Can you work these out from the model? Positions are in its coordinate system, mm. Face numbers are marked on the shaded views. A direction names the side the tool comes from. Give positions to 0.01 mm unless a question says otherwise; leave off trailing zeros. Order: outer loops, then holes, each group sorted by start corner. A loop starts at its lowest first (then second) coordinate and runs counter-clockwise, first axis right, second up.
Item 1: I want a section at A-A, the plane x = 9. Write out the boundary of the cut face in (y, z).
Item 2: I'm going to push flat-ended pins straight in: pin 1 Ø4 at (y, z) = (9.5, 48.5) entering from +X; pin 2 Ø3 at (y, z) = (9.5, 12) entering from +X; pin 3 Ø8 at (y, z) = (9, 37) entering from +X. Where does each tip first touch, or does it pass through?
Item 3: I want a section at C-C, the plane z = 34. Write out the boundary of the cut face in (x, y), then the cut area to 3 significant figures.
Item 4: If I drill on line 1 along X through (y, z) = (-23.85, 2.5); line 2 along Z through (x, y) = (-9, -23.9); line 3 along Y through (x, z) = (-7, 44.5), over which ranges is the centre line in solid material (lowest first)?
Item 5: If we mould it in two halves opening along Y, with no side actions, what happens to the marked faces 1, 2 and 3? For each: +Y half, -Y half, draft (parallel to the pull), parting line (faces both ways), or undercut.
Item 6: I want a section at B-B, the plane z = 2.5. Count the separate pieces of the cut face and the enclosed holes in it, then the cut area to 3 significant figures.
Item 7: Which directions (+Z, -Z, +X, -X, +Y, -Y) give clear straight access to the entire face, cutting with the end or side of a thin tool? Please do the marked faces 4 and 5.
Item 8: I want a section at D-D, the plane y = 19. Write out the boundary of the cut face in (x, z).
Autodesk Inventor part; units mm, degrees
ref_plane "YZ Plane" through (0, 0, 0) normal (1, 0, 0) x (0, 1, 0)
ref_plane "XZ Plane" through (0, 0, 0) normal (0, 1, 0) x (-1, 0, 0)
ref_plane "XY Plane" through (0, 0, 0) normal (0, 0, 1) x (1, 0, 0)
sketch "Sketch1" plane through (0, 0, 0) normal (0, 0, 1) x (1, 0, 0)
  circle A0 centre (0, 0) radius 28.8
  line L0 (-50, 23.8) -> (50, 23.8)
  line L1 (50, 23.8) -> (50, -23.8)
  line L2 (50, -23.8) -> (-50, -23.8)
  line L3 (-50, -23.8) -> (-50, 23.8)
  point P0 (50, 0)
  point P1 (0, 23.8)
  point P2 (-16.217275, -23.8)
  point P3 (16.217275, -23.8)
  point P4 (16.217275, 23.8)
  point P5 (-16.217275, 23.8)
  dimension "d0" = 57.6
  dimension "d1" = 47.6
  dimension "d2" = 100
sketch "Sketch1 outline for Extrusion1" plane through (0, 0, 0) normal (0, 0, 1) x (1, 0, 0)
  line L0 (-16.217275, -23.8) -> (16.217275, -23.8)
  arc A0 (-16.217275, 23.8) -> (-16.217275, -23.8) centre (0, 0) ccw
  line L1 (16.217275, 23.8) -> (-16.217275, 23.8)
  arc A1 (16.217275, -23.8) -> (16.217275, 23.8) centre (0, 0) ccw
extrude "Extrusion1" add sketch "Sketch1 outline for Extrusion1" along normal blind 80
fillet "Fillet1" radius 1 4 edges at (-16.2173, 23.8, 40) (16.2173, 23.8, 40) (16.2173, -23.8, 40) (-16.2173, -23.8, 40)
thicken "Thicken1" operation add thickness 0.2 both sides no extend neighbours no toward (0, 1, 0) faces at (5.301991, 23.8, 26.666667) (-16.040924, 23.790852, 26.666667) (-27.332956, -9.074665, 53.333333) (16.237959, 23.743284, 26.666667) (28.430873, 4.596242, 53.333333) (16.362219, -23.689854, 26.666667) (-5.301991, -23.8, 26.666667) (-16.362219, -23.689854, 26.666667)
shell "Shell1" thickness 0.2 removed faces 2 at (-5.301991, -8, 80) at (-5.301991, -8, 0)
sketch "Sketch2" plane through (-19.580613, 24, 0) normal (0, 1, 0) x (1, 0, 0)
  line L0 (10.580613, -2.5) -> (28.580613, -2.5) construction
  line L1 (35.486587, 0) -> (3.674639, 0)
  point P0 (19.580613, 0)
  point P1 (31.432467, 0)
  point P2 (0, 0)
  point P3 (19.580613, -2.5)
  point P4 (19.580613, 0)
  point P5 (27.757828, 0)
  point P6 (19.580613, 0)
  dimension "d9" = 18
  dimension "d10" = 2.5
hole "Hole1" at (-9, 24, 2.5) at (9, 24, 2.5) direction (0, -1, 0) diameter 2.1 end through all
equation "\"d0\" = phi + 2 * slack"
equation "\"d1\" = flat_width + 2 * slack"
equation "\"flat_width\" = 44"
equation "\"phi\" = 54"
equation "\"slack\" = 1.8"
properties part number "probe-side-large-mesh" material "Stainless Steel"
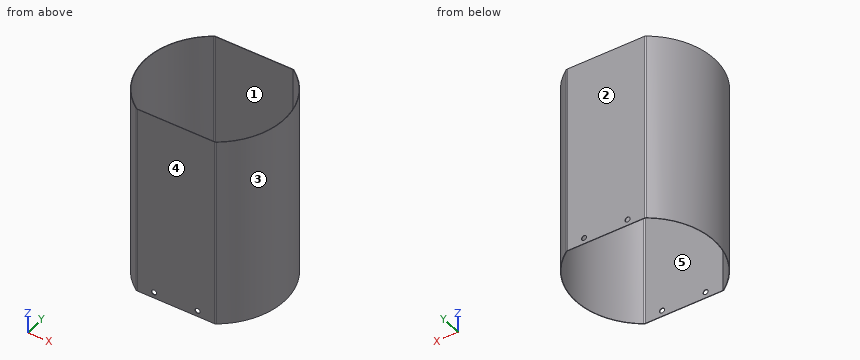
Results list:
1. outline: (-24, 0) - (-23.8, 0) - (-23.8, 1.45) - (-24, 1.45) - close; (-24, 3.55) - (-23.8, 3.55) - (-23.8, 80) - (-24, 80) - close; (23.8, 0) - (24, 0) - (24, 1.45) - (23.8, 1.45) - close; (23.8, 3.55) - (24, 3.55) - (24, 80) - (23.8, 80) - close
2. pin 1: stops at x = 28.01
2. pin 2: stops at x = 27.87
2. pin 3: stops at x = 28.57
3. outline: (-16.59, -23.78) arc R1.2 ccw to (-15.91, -24) - (15.91, -24) arc R1.2 ccw to (16.59, -23.78) arc R29 ccw to (16.59, 23.78) arc R1.2 ccw to (15.91, 24) - (-15.91, 24) arc R1.2 ccw to (-16.59, 23.78) arc R29 ccw to start; hole (-16.48, -23.62) arc R1 ccw to (-15.91, -23.8) - (15.91, -23.8) arc R1 ccw to (16.48, -23.62) arc R28.8 ccw to (16.48, 23.62) arc R1 ccw to (15.91, 23.8) - (-15.91, 23.8) arc R1 ccw to (-16.48, 23.62) arc R28.8 ccw to start
3. area: 35.5 mm2
4. line 1: x = -16.49 to -10.05, -7.95 to 7.95, 10.05 to 16.49
4. line 2: z = 0 to 1.45, 3.55 to 80
4. line 3: y = -24 to -23.8, 23.8 to 24
5. face 1: undercut
5. face 2: +Y half
5. face 3: parting line
6. separate pieces: 4
6. enclosed holes: 0
6. area: 33.8 mm2
7. face 4: +Z, -Z, +X, -X, -Y
7. face 5: +Z, -Z
8. outline: (-21.91, 0) - (-21.64, 0) - (-21.64, 80) - (-21.91, 80) - close; (21.64, 0) - (21.91, 0) - (21.91, 80) - (21.64, 80) - close
